from build123d import *

# Parameters (mm, degrees)
F0_W      = 41
F0_H      = 57
F1_DEPTH  = 34
F2_W      = 35
F2_H      = 57
F3_DEPTH  = 31.5
F5_DEPTH  = 41.001
F6_R      = 1
F7_DEPTH  = 41.001
F8_W      = 3
F8_H      = 5
F8_W_2    = 5
F8_H_2    = 2.5
F9_DEPTH  = 2.5
F10_W     = 5
F10_H     = 13
F11_DEPTH = 4


with BuildPart() as f1:
    # F0 (on Top) → F1 (new body)
    with BuildSketch(Plane.XY):
        with Locations((-3.310106, 5.843145)):
            Rectangle(F0_W, F0_H)
    extrude(amount=F1_DEPTH)

    # F2 (on face) → F3 (cut)
    with BuildSketch(Plane.XY.offset(34)):
        with Locations((-3.310106, 5.843145)):
            Rectangle(F2_W, F2_H)
    extrude(amount=-F3_DEPTH, mode=Mode.SUBTRACT)

    # F4 (on face) → F5 (cut, through all)
    with BuildSketch(Plane.YZ.offset(17.189894)):
        with BuildLine():
            ThreePointArc((-22.656855, 2.5), (1.780705, 25.601082), (34.343145, 34))
            Line((34.343145, 34), (-22.656855, 34))
            Line((-22.656855, 34), (-22.656855, 2.5))
        make_face()
    extrude(amount=-F5_DEPTH, mode=Mode.SUBTRACT)

    # F6 (on face) → F7 (cut, through all)
    with BuildSketch(Plane.YZ.offset(17.189894)):
        with Locations((-20.156855, 3.5)):
            Circle(F6_R)
    extrude(amount=-F7_DEPTH, mode=Mode.SUBTRACT)

    # F8 (on face) → F9 (cut)
    with BuildSketch(Plane(origin=(0, 34.343145, 0), x_dir=(-1, 0, 0), z_dir=(0, 1, 0))):
        with Locations((-15.689894, 17)):
            Rectangle(F8_W, F8_H)
        with Locations((3.310106, 1.25)):
            Rectangle(F8_W_2, F8_H_2)
        with Locations((22.310106, 17)):
            Rectangle(F8_W, F8_H)
    extrude(amount=-F9_DEPTH, mode=Mode.SUBTRACT)

    # F10 (on face) → F11 (join)
    with BuildSketch(Plane(origin=(0, 0, 0), x_dir=(1, 0, 0), z_dir=(0, 0, -1))):
        with Locations((14.689894, -1.843145)):
            Rectangle(F10_W, F10_H)
        with Locations((-21.310106, -1.843145)):
            Rectangle(F10_W, F10_H)
    extrude(amount=F11_DEPTH)


solid = f1.part
Design review of the part built by this model. Coordinates are the model's own, in mm. A direction names the side the tool comes from. Round coordinates to 2 decimals unless told otherwise and drop trailing zeros. Order: outer loops, then holes, each group sorted by start corner. A loop starts at its lowest first (then second) coordinate and runs counter-clockwise, first axis right, second up.
1) Draft analysis for pull direction Z (two halves, no side actions). For faces 6 (the cylindrical face through (-22.289, -21.156, 3.544)), 7 (the flat face through (-21, 2, -4)), 8 (the flat face through (-0.81, 33, 1)), state which applies: released by +Z, released by -Z, zero draft, split by the parting line, or undercut.
The answers:
face 6: undercut
face 7: released by -Z
face 8: zero draft
2) Clearance check with flat-ended pins moving along their axes: pin 1 Ø2 at (x, y) = (-22, 33) entering from +Z; pin 2 Ø8 at (x, y) = (7.5, -3) entering from -Z; pin 3 Ø6 at (x, y) = (-1, 19) entering from +Z. State where each tip first meets the part, or that it passes through.
The answers:
pin 1: stops at z = 34
pin 2: stops at z = 0
pin 3: stops at z = 2.5
3) Machinability: for faces 1 (the flat face through (-18.81, 2, -2)), 2 (the flat face through (16, 33, 14.5)), 3 (the flat face through (15, -4.657, -2)), 4 (the flat face through (-3, 31.843, 1)), 5 (the flat face through (14.19, 12, 15)), which of the approach directions +Z, -Z, +X, -X, +Y, -Y give a long, thin tool a straight path to every point of the face, cutting with its end or side? Answer none if there is none.
The answers:
face 1: -Z, +Y, -Y
face 2: +X, -X, +Y
face 3: -Z, +X, -X, -Y
face 4: +Z, -Z, +Y
face 5: +Z, +Y, -Y
4) Consider section B-B (z = 3.5). State the section outline as (x, y) points.
The answers:
outline: (-23.81, -22.02) - (-20.81, -22.02) - (-20.81, -21.16) - (-23.81, -21.16) - close; (-23.81, -19.16) - (-20.81, -19.16) - (-20.81, 34.34) - (-23.81, 34.34) - close; (14.19, -22.02) - (17.19, -22.02) - (17.19, -21.16) - (14.19, -21.16) - close; (14.19, -19.16) - (17.19, -19.16) - (17.19, 34.34) - (14.19, 34.34) - close
5) Consider section D-D (x = -14). State the section outline as (y, z) points, plus the area to 4 significant figures.
The answers:
outline: (-22.66, 0) - (34.34, 0) - (34.34, 2.5) - (-22.66, 2.5) - close
area: 142.5 mm2
6) Consider section C-C (y = 19.5). State the section outline as (x, z) points, plus the area to 3 significant figures.
The answers:
outline: (-23.81, 0) - (17.19, 0) - (17.19, 32.34) - (14.19, 32.34) - (14.19, 2.5) - (-20.81, 2.5) - (-20.81, 32.34) - (-23.81, 32.34) - close
area: 282 mm2
7) Consider section A-A (z = 16). State the section outline as (x, y) points, plus the area to 3 significant figures.
The answers:
outline: (-23.81, -11.48) - (-20.81, -11.48) - (-20.81, 31.84) - (-23.81, 31.84) - close; (14.19, -11.48) - (17.19, -11.48) - (17.19, 31.84) - (14.19, 31.84) - close
area: 260 mm2
8) For L1, parallel to X at y = 18, z = 13; L2, parallel to Z at x = -11, y = 7; L3, parallel to Y at x = 16.35, z = 3.5, list the stretches that pass through material, from the lowest coordinate up.
The answers:
L1: x = -23.81 to -20.81, 14.19 to 17.19
L2: z = 0 to 2.5
L3: y = -22.02 to -21.16, -19.16 to 34.34
